Part print with two shaded views. Sizes in mm from the minimum x, y, z corner. Give positions to 0.01 mm unless a question says otherwise; leave off trailing zeros. Write each loop counter-clockwise with the first axis right and the second up, starting at its lowest first coordinate (ties: lowest second). Pieces come first, ordered by that corner, then holes.
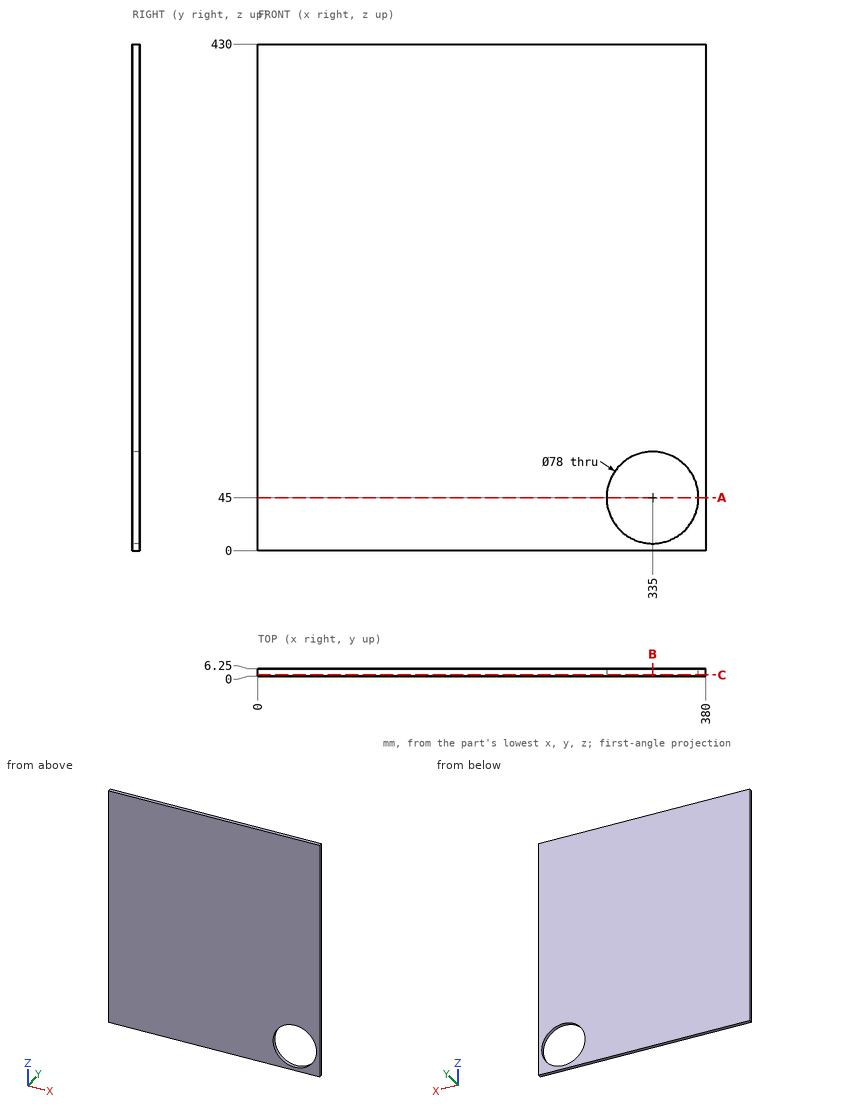
1) Drill centre lines: L1, parallel to Z at x = 335, y = 4.75; L2, parallel to X at y = 1, z = 28. Where is each one in solid material? Low to high.
Check result:
L1: z = 0 to 6, 84 to 430
L2: x = 0 to 299.9, 370.1 to 380
2) Saw through at C-C (y = 1). Write the cut outline in (x, z).
Check result:
outline: (0, 0) - (380, 0) - (380, 430) - (0, 430) - close; hole circle Ø78 at (335, 45)
3) Saw through at A-A (z = 45). Write the cut outline in (x, y).
Check result:
outline: (0, 0) - (296, 0) - (296, 6.25) - (0, 6.25) - close; (374, 0) - (380, 0) - (380, 6.25) - (374, 6.25) - close
4) Saw through at B-B (x = 335). Write the cut outline in (y, z), and give its area (3 significant figures).
Check result:
outline: (0, 0) - (6.25, 0) - (6.25, 6) - (0, 6) - close; (0, 84) - (6.25, 84) - (6.25, 430) - (0, 430) - close
area: 2,200 mm2
